Input: part model. Units: mm. Frame: model coordinates. A direction names the side the tool comes from. Give positions to 0.01 mm unless a question says otherwise; leave off trailing zeros. Write each loop counter-clockwise with the first axis right and the second up, starting at its lowest first coordinate (ties: lowest second). Pieces come first, ordered by that corner, then holes.
```python
from build123d import *

# Parameters (mm, degrees)
F0_W      = 212
F0_H      = 221
F1_DEPTH  = 201
F2_W      = 206
F2_H      = 112
F3_DEPTH  = 198
F4_W      = 212
F4_H      = 144
F5_DEPTH  = 100
F2_H_2    = 3
F6_DEPTH  = 54
F2_H_3    = 100
F7_DEPTH  = 54
F9_DEPTH  = 6
F11_START = 198
F10_W     = 220
F10_H     = 228
F10_W_2   = 206
F10_H_2   = 112
F11_DEPTH = 105
F14_DEPTH = 109.5


with BuildPart() as f1:
    # F0 (on Top) → F1 (new body)
    with BuildSketch(Plane.XY):
        Rectangle(F0_W, F0_H)
    extrude(amount=F1_DEPTH)

    # F2 (on face) → F3 (cut)
    with BuildSketch(Plane.XY.offset(201)):
        with Locations((0, 51.5)):
            Rectangle(F2_W, F2_H)
    extrude(amount=-F3_DEPTH, mode=Mode.SUBTRACT)

    # F4 (on face) → F5 (cut)
    with BuildSketch(Plane.XZ.offset(110.5)):
        with Locations((0, 72)):
            Rectangle(F4_W, F4_H)
    extrude(amount=-F5_DEPTH, mode=Mode.SUBTRACT)

    # F2 (on face) → F6 (cut)
    with BuildSketch(Plane.XY.offset(201)):
        with Locations((0, -6)):
            Rectangle(F2_W, F2_H_2)
    extrude(amount=-F6_DEPTH, mode=Mode.SUBTRACT)

    # F2 (on face) → F7 (cut)
    with BuildSketch(Plane.XY.offset(201)):
        with Locations((0, -57.5)):
            Rectangle(F2_W, F2_H_3)
    extrude(amount=-F7_DEPTH, mode=Mode.SUBTRACT)

    # F8 (on face) → F9 (cut, through all)
    with BuildSketch(Plane.XZ.offset(10.5)):
        with BuildLine():
            Line((-28.3372546306, 42.5), (28.3372546306, 42.5))
            ThreePointArc((28.3372546306, 42.5), (42, 73.5), (28.3372546306, 104.5))
            Line((28.3372546306, 104.5), (-28.3372546306, 104.5))
            ThreePointArc((-28.3372546306, 104.5), (-42, 73.5), (-28.3372546306, 42.5))
        make_face()
        with BuildLine():
            Line((56, 104.5), (56, 101.25))
            ThreePointArc((56, 101.25), (58.2980970389, 102.2019029611), (59.25, 104.5))
            ThreePointArc((59.25, 104.5), (56, 107.75), (52.75, 104.5))
            Line((52.75, 104.5), (56, 104.5))
        make_face()
        with BuildLine():
            ThreePointArc((52.75, 104.5), (53.7019029611, 102.2019029611), (56, 101.25))
            Line((56, 101.25), (56, 104.5))
            Line((56, 104.5), (52.75, 104.5))
        make_face()
        with BuildLine():
            ThreePointArc((56, 45.75), (53.7019029611, 44.7980970389), (52.75, 42.5))
            Line((52.75, 42.5), (56, 42.5))
            Line((56, 42.5), (56, 45.75))
        make_face()
        with BuildLine():
            Line((56, 42.5), (52.75, 42.5))
            ThreePointArc((52.75, 42.5), (56, 39.25), (59.25, 42.5))
            ThreePointArc((59.25, 42.5), (58.2980970389, 44.7980970389), (56, 45.75))
            Line((56, 45.75), (56, 42.5))
        make_face()
        with BuildLine():
            ThreePointArc((-56, 45.75), (-58.2980970389, 40.2019029611), (-52.75, 42.5))
            Line((-52.75, 42.5), (-56, 42.5))
            Line((-56, 42.5), (-56, 45.75))
        make_face()
        with BuildLine():
            Line((-56, 42.5), (-52.75, 42.5))
            ThreePointArc((-52.75, 42.5), (-53.7019029611, 44.7980970389), (-56, 45.75))
            Line((-56, 45.75), (-56, 42.5))
        make_face()
        with BuildLine():
            Line((-56, 104.5), (-56, 101.25))
            ThreePointArc((-56, 101.25), (-53.7019029611, 102.2019029611), (-52.75, 104.5))
            Line((-52.75, 104.5), (-56, 104.5))
        make_face()
        with BuildLine():
            ThreePointArc((-52.75, 104.5), (-58.2980970389, 106.7980970389), (-56, 101.25))
            Line((-56, 101.25), (-56, 104.5))
            Line((-56, 104.5), (-52.75, 104.5))
        make_face()
    extrude(amount=-F9_DEPTH, mode=Mode.SUBTRACT)

    # F10 (on face) → F11 (join)
    with BuildSketch(Plane.XY.offset(3).offset(F11_START)):
        Rectangle(F10_W, F10_H)
        with Locations((0, 51.5)):
            Rectangle(F10_W_2, F10_H_2, mode=Mode.SUBTRACT)
    extrude(amount=F11_DEPTH)

    # F13 (on face) → F14 (cut, through all)
    with BuildSketch(Plane.XZ.offset(114)):
        Polygon((1, 289), (-56, 289), (-56, 240), (87, 240), (87, 272), align=None)
    extrude(amount=-F14_DEPTH, mode=Mode.SUBTRACT)


solid = f1.part
```
Q1. Mould query, pull axis X, two halves, no side actions, for faces 6 (the flat face through (-106.4, 0.5, 201)), 7 (the flat face through (110, -2, 253)), 8 (the flat face through (44.6, -60.02, 280.38)). Classes: +X half, -X half, draft (parallel to the pull), parting line (faces both ways), or undercut.
Q2. Section B-B, the plane y = -74. Return the cut outline in (x, z), then the cut area to 3 significant figures.
Q3. Material intervals for line 1 along X through (y, z) = (-6, 42); line 2 along Z through (x, y) = (-2.5, -90); line 3 along X through (y, z) = (32, 27), sorted ascending.
Q4. Access query for faces 1 (the flat face through (-56, -60, 265)), 2 (the flat face through (-1, -10.5, 41)), 3 (the flat face through (-1, 110.5, 99)), 4 (the flat face through (-1, -107.5, 174)), 5 (the flat face through (-1, 107.5, 152)). Directions: +Z, -Z, +X, -X, +Y, -Y. A direction counts if a zero-diameter tool reaches every point of the face in a straight line with its end or side. Return the directions, or none.
Q5. Section D-D, the plane z = 181. Return the cut outline in (x, y), then the cut area to 3 significant figures.
Q6. Section A-A, the plane x = -4.5. Return the cut outline in (y, z), then the cut area to 3 significant figures.
Q7. Section C-C, the plane y = 13. Return the cut outline in (x, z).
Q8. Pin query (flat end, axial travel): pin 1 (12 mm diameter, centred on x = 88, z = 152.5, fed in from +Y); pin 2 (17 mm diameter, centred on x = 41, z = 163, fed in from -Y); pin 3 (3 mm diameter, centred on x = 22.5, z = 32.5, fed in from -Y); pin 4 (1.8 mm diameter, centred on x = 3, y = -9, fed in from -Z). Return the tip coordinate at first contact, or that it passes through.
Solutions:
1. face 6: draft
1. face 7: +X half
1. face 8: undercut
2. outline: (-110, 201) - (-106, 201) - (-106, 144) - (106, 144) - (106, 201) - (110, 201) - (110, 306) - (-110, 306) - close; hole (-103, 147) - (103, 147) - (103, 201) - (-103, 201) - close; hole (-56, 240) - (87, 240) - (87, 272) - (1, 289) - (-56, 289) - close
2. area: 17,800 mm2
3. line 1: x = -106 to -59.21, -52.79 to 52.79, 59.21 to 106
3. line 2: z = 144 to 147, 201 to 240, 289 to 306
3. line 3: x = -106 to -103, 103 to 106
4. face 1: -Y
4. face 2: -Z, +X, -X, -Y
4. face 3: -Z, +X, -X, +Y
4. face 4: none
4. face 5: +Z
5. outline: (-106, -110.5) - (106, -110.5) - (106, 110.5) - (-106, 110.5) - close; hole (-103, -107.5) - (103, -107.5) - (103, 107.5) - (-103, 107.5) - close
5. area: 2,560 mm2
6. outline: (-114, 201) - (-110.5, 201) - (-110.5, 144) - (-10.5, 144) - (-10.5, 104.5) - (-4.5, 104.5) - (-4.5, 147) - (-107.5, 147) - (-107.5, 201) - (-4.5, 201) - (-4.5, 240) - (-114, 240) - close; (-114, 289) - (-4.5, 289) - (-4.5, 306) - (-114, 306) - close; (-10.5, 0) - (110.5, 0) - (110.5, 201) - (114, 201) - (114, 306) - (107.5, 306) - (107.5, 3) - (-4.5, 3) - (-4.5, 42.5) - (-10.5, 42.5) - close
6. area: 8,730 mm2
7. outline: (-110, 201) - (-106, 201) - (-106, 0) - (106, 0) - (106, 201) - (110, 201) - (110, 306) - (103, 306) - (103, 3) - (-103, 3) - (-103, 306) - (-110, 306) - close
8. pin 1: stops at y = 110.5
8. pin 2: stops at y = -110.5
8. pin 3: stops at y = -10.5
8. pin 4: stops at z = 0
